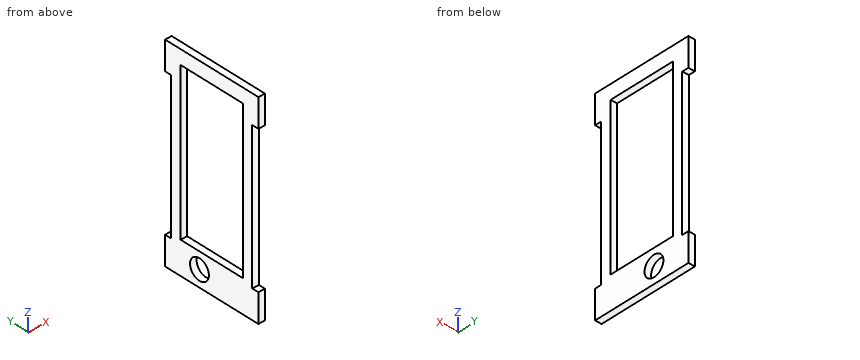
Autodesk Inventor part; units mm, degrees
ref_plane "YZ Plane" through (0, 0, 0) normal (1, 0, 0) x (0, 1, 0)
ref_plane "XZ Plane" through (0, 0, 0) normal (0, 1, 0) x (-1, 0, 0)
ref_plane "XY Plane" through (0, 0, 0) normal (0, 0, 1) x (1, 0, 0)
sketch "Sketch1" plane through (0, 0, 0) normal (1, 0, 0) x (0, 1, 0)
  line L0 (-92.7646, -8.503) -> (-89.7646, -8.503)
  line L1 (-89.7646, -8.503) -> (-89.7646, -11.753)
  line L2 (-89.7646, -11.753) -> (-92.7646, -11.753)
  line L3 (-92.7646, -11.753) -> (-92.7646, -8.503)
  line L4 (-92.7646, -21.6527) -> (-89.7646, -21.6527)
  line L5 (-89.7646, -21.6527) -> (-89.7646, -21.7527)
  line L6 (-89.7646, -21.7527) -> (-92.7646, -21.7527)
  line L7 (-92.7646, -21.7527) -> (-92.7646, -21.6527)
  line L8 (-21.5, 50) -> (21.5, 50)
  line L9 (21.5, 50) -> (21.5, -50)
  line L10 (21.5, -50) -> (-21.5, -50)
  line L11 (-21.5, -50) -> (-21.5, 50)
  line L12 (0, 50) -> (0, -50) construction
  line L13 (-21.5, 0) -> (21.5, 0) construction
  line L14 (-16.5, 43) -> (16.5, 43)
  line L15 (16.5, 43) -> (16.5, -34)
  line L16 (16.5, -34) -> (-16.5, -34)
  line L17 (-16.5, -34) -> (-16.5, 43)
  circle A0 centre (6.5, -42) radius 5
  line L18 (-21.5, 50) -> (-24.75, 50)
  line L19 (-24.75, 50) -> (-24.75, 36)
  line L20 (-24.75, 36) -> (-21.5, 36)
  line L21 (-21.5, 36) -> (-21.5, 50)
  line L22 (21.5, 50) -> (24.75, 50)
  line L23 (24.75, 50) -> (24.75, 36)
  line L24 (24.75, 36) -> (21.5, 36)
  line L25 (21.5, 36) -> (21.5, 50)
  line L26 (-21.5, -50) -> (-24.75, -50)
  line L27 (-24.75, -50) -> (-24.75, -36)
  line L28 (-24.75, -36) -> (-21.5, -36)
  line L29 (-21.5, -36) -> (-21.5, -50)
  line L30 (21.5, -36) -> (21.5, -50)
  line L31 (24.75, -50) -> (24.75, -36)
  line L32 (24.75, -36) -> (21.5, -36)
  line L33 (21.5, -50) -> (24.75, -50)
  point P0 (0, 0)
  dimension "d0" = 3
  dimension "mat" = 3.25
  dimension "d2" = 3
  dimension "kerf" = 0.1
  dimension "d4" = 43
  dimension "d5" = 100
  dimension "d9" = 7
  dimension "d10" = 16
  dimension "d11" = 5
  dimension "d12" = 5
  dimension "d13" = 10
  dimension "d15" = 3
  dimension "d16" = 3.25
  dimension "d17" = 14
  dimension "d24" = 10
extrude "Extrusion1" [suppressed]
extrude "Extrusion2" add sketch "Sketch1" along normal blind 3.25 contours L11 L20 L19 L18 | L22 L23 L24 L9 | L11 L26 L27 L28 | L32 L31 L33 L9
extrude "Extrusion3" add sketch "Sketch1" along normal blind 3.25 contours L8 L9 L10 L11
equation "\"d16\" = mat"
equation "\"d18\" = mat"
equation "\"d20\" = mat"
equation "\"d22\" = mat"
properties part number "body-side2"
Part model, mm, in its own coordinate system. Round coordinates to 2 decimals unless told otherwise and drop trailing zeros. Loops run counter-clockwise (first coordinate to the right, second up) from the corner with the lowest first, then second, coordinate; pieces in that order, holes last. Notation, with made-up numbers: (70.25, 33.25) -> (127.25, 33.25) arc R23 ccw to (127.25, 62.25) -> close; hole circle Ø6 at (88.25, -11.5). An arc over 180 degrees is marked (long way). Use CSV: the item, a comma, the result in double quotes. Start each with the question number.
1) Cut at A-A, the plane z = -42. Write the cut outline in (x, y).
2) Drop flat-ended pins along their axis: P1, Ø6, axis at y = 6.5, z = -42, coming from the -X side; P2, Ø5, axis at y = 19, z = 16.5, coming from the -X side; P3, Ø1.6, axis at x = 2, z = -9, coming from the -Y side; P4, Ø1, axis at x = 3, z = 27, coming from the +Y side. Give the stop position or say it passes through.
3) Cut at B-B, the plane y = -14. Write the cut outline in (x, z), plus the area to 4 significant figures.
4) Cut at C-C, the plane y = 6.5. Write the cut outline in (x, z).
5) Cut at D-D, the plane x = 2.25. Write the cut outline in (y, z).
6) Wall check: L1, parallel to Z at x = 2.1, y = 6.5; L2, parallel to Z at x = 2.45, y = 13.5; L3, parallel to Z at x = 1.5, y = -22. Give the ranges that are in metal, low to high. Write a range as [from, to].
Determined:
1,outline,"(0, -24.75) -> (3.25, -24.75) -> (3.25, 1.5) -> (0, 1.5) -> close; (0, 11.5) -> (3.25, 11.5) -> (3.25, 24.75) -> (0, 24.75) -> close"
2,P1,"passes through"
2,P2,"stops at x = 0"
2,P3,"stops at y = -21.5"
2,P4,"stops at y = 21.5"
3,outline,"(0, -50) -> (3.25, -50) -> (3.25, -34) -> (0, -34) -> close; (0, 43) -> (3.25, 43) -> (3.25, 50) -> (0, 50) -> close"
3,area,"74.75 mm2"
4,outline,"(0, -50) -> (3.25, -50) -> (3.25, -47) -> (0, -47) -> close; (0, -37) -> (3.25, -37) -> (3.25, -34) -> (0, -34) -> close; (0, 43) -> (3.25, 43) -> (3.25, 50) -> (0, 50) -> close"
5,outline,"(-24.75, -50) -> (24.75, -50) -> (24.75, -36) -> (21.5, -36) -> (21.5, 36) -> (24.75, 36) -> (24.75, 50) -> (-24.75, 50) -> (-24.75, 36) -> (-21.5, 36) -> (-21.5, -36) -> (-24.75, -36) -> close; hole (-16.5, -34) -> (16.5, -34) -> (16.5, 43) -> (-16.5, 43) -> close; hole circle Ø10 at (6.5, -42)"
6,L1,"z = [-50, -47], [-37, -34], [43, 50]"
6,L2,"z = [-50, -34], [43, 50]"
6,L3,"z = [-50, -36], [36, 50]"
